Work out the finished part from the listing and answer in its coordinate system (mm). Face numbers are marked on the shaded views. A direction names the side the tool comes from. Round coordinates to 2 decimals unless told otherwise and drop trailing zeros. Loops run counter-clockwise (first coordinate to the right, second up) from the corner with the lowest first, then second, coordinate; pieces in that order, holes last. Notation, with made-up numbers: (-35, 31) - (-3, 31) arc R18 ccw to (-3, 40) - close; hole circle Ø1 at (-16, 66.25). An arc over 180 degrees is marked (long way). Use CSV: the item, a comma, the result in double quotes. Start each with the question number.
from build123d import *

# Parameters (mm, degrees)
SKETCH1_R           = 1
BOSS_EXTRUDE1_DEPTH = 1.5
CIRPATTERN1_COUNT   = 4
SKETCH3_R           = 2.525
SKETCH3_R_2         = 1.525
BOSS_EXTRUDE3_DEPTH = 7.25


with BuildPart() as part:
    # Sketch1 → Boss-Extrude1 (new body)
    with BuildSketch(Plane.XY):
        with BuildLine():
            Line((1.8, 2.706011826), (1.8, 9.915))
            ThreePointArc((1.8, 9.915), (0, 11.715), (-1.8, 9.915))
            Line((-1.8, 9.915), (-1.8, 2.706011826))
            ThreePointArc((-1.8, 2.706011826), (0, -3.25), (1.8, 2.706011826))
        make_face()
        with Locations((0, 5.015)):
            Circle(SKETCH1_R, mode=Mode.SUBTRACT)
        with Locations((0, 9.915)):
            Circle(SKETCH1_R, mode=Mode.SUBTRACT)
    boss_extrude1 = extrude(amount=BOSS_EXTRUDE1_DEPTH)

    # CirPattern1: Boss-Extrude1 ×4 about axis
    cirpattern1_axis = Axis((0, 0, 0), (0, 0, 1))
    for i in range(1, CIRPATTERN1_COUNT):
        add(boss_extrude1.rotate(cirpattern1_axis, i * 360 / CIRPATTERN1_COUNT))

    # Sketch3 → Boss-Extrude3 (add)
    # profile 1 of 3: a face of its own
    with BuildSketch(Plane.XY.offset(1.5)):
        with Locations(Location((0, 0, 0), (0, 0, 180))):
            Circle(SKETCH3_R)
        Circle(SKETCH3_R_2, mode=Mode.SUBTRACT)
    # profile 2 of 3: a face of its own
    with BuildSketch(Plane.XY.offset(1.5)):
        with BuildLine():
            ThreePointArc((1.129158979, 1.025), (0, 1.525), (-1.129158979, 1.025))
            Line((-1.129158979, 1.025), (1.129158979, 1.025))
        make_face()
    # profile 3 of 3: a face of its own
    with BuildSketch(Plane.XY.offset(1.5)):
        with BuildLine():
            ThreePointArc((1.129158979, 1.025), (0, 1.525), (-1.129158979, 1.025))
            Line((-1.129158979, 1.025), (1.129158979, 1.025))
        make_face()
    extrude(amount=BOSS_EXTRUDE3_DEPTH)


solid = part.part
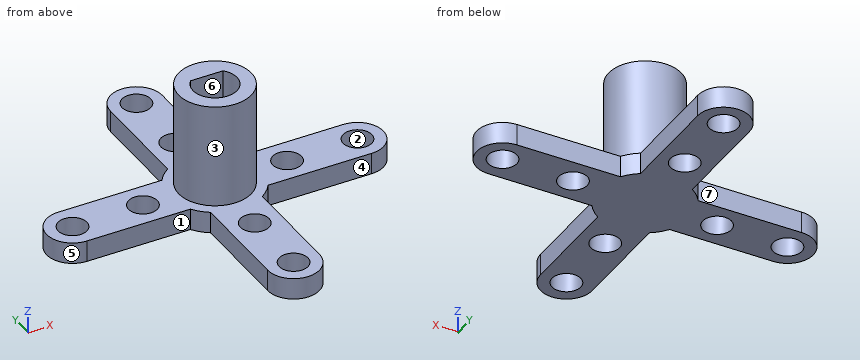
Item 1: The mould has two halves that part along Y. Classify the marked faces 5, 6 and 7: pulls with the +Y half, pulls with the -Y half, needs draft (parallel to the pull), parting line crosses it, or undercut.
Item 2: A cutting plane is placed at D-D (z = 2.5). Determine the outline of the cut face in (x, y) (3 decimals), plus the area to 3 significant figures.
Item 3: Each of these flat-tipped pins is pushed along its axis until it touches: pin 1 Ø1.6 at (x, z) = (-6, 0.5) entering from +Y; pin 2 Ø1.2 at (x, y) = (5.015, 0) entering from +Z; pin 3 Ø2.5 at (x, y) = (0, 0) entering from -Z; pin 4 Ø1.6 at (y, z) = (-7.5, 1) entering from -X. Where does it stop, or does it pass through?
Item 4: Find the intervals of material crossed by probe 1 along Y at (x, z) = (0, 1.05) (3 decimals); probe 2 along Z at (x, y) = (1.5, -9.5), in increasing order. Write a range as [from, to].
Item 5: A cutting plane is placed at A-A (y = 0). Determine the outline of the cut face in (x, z) (3 decimals), plus the area to 3 significant figures.
Item 6: A cutting plane is placed at C-C (y = 5.5). Determine the outline of the cut face in (x, z).
Item 7: Which of the six approach directions +Z, -Z, +X, -X, +Y, -Y give full straight-line access (tool end or side, diameter ignored) to the marked faces 1, 2, 3 and 4?
Item 8: A cutting plane is placed at B-B (x = 0). Determine the outline of the cut face in (y, z) (3 decimals), plus the area to 3 significant figures.
Result sheet:
1,face 5,"parting line crosses it"
1,face 6,"undercut"
1,face 7,"pulls with the +Y half"
2,outline,"circle Ø5.05 at (0, 0); hole (-1.129, 1.025) arc R1.525 ccw (long way) to (1.129, 1.025) - close"
2,area,"13.5 mm^2"
3,pin 1,"y = 1.8"
3,pin 2,"through"
3,pin 3,"z = 0"
3,pin 4,"x = -1.8"
4,probe 1,"[-11.715, -10.915], [-8.915, -6.015], [-4.015, 4.015], [6.015, 8.915], [10.915, 11.715]"
4,probe 2,"[0, 1.5]"
5,outline,"(-11.715, 0) - (-10.915, 0) - (-10.915, 1.5) - (-11.715, 1.5) - close; (-8.915, 0) - (-6.015, 0) - (-6.015, 1.5) - (-8.915, 1.5) - close; (-4.015, 0) - (4.015, 0) - (4.015, 1.5) - (2.525, 1.5) - (2.525, 8.75) - (1.525, 8.75) - (1.525, 1.5) - (-1.525, 1.5) - (-1.525, 8.75) - (-2.525, 8.75) - (-2.525, 1.5) - (-4.015, 1.5) - close; (6.015, 0) - (8.915, 0) - (8.915, 1.5) - (6.015, 1.5) - close; (10.915, 0) - (11.715, 0) - (11.715, 1.5) - (10.915, 1.5) - close"
5,area,"37.6 mm^2"
6,outline,"(-1.8, 0) - (-0.87, 0) - (-0.87, 1.5) - (-1.8, 1.5) - close; (0.87, 0) - (1.8, 0) - (1.8, 1.5) - (0.87, 1.5) - close"
7,face 1,"+Z, -Z, -X, -Y"
7,face 2,"+Z, -Z"
7,face 3,"+Z"
7,face 4,"+Z, -Z, +X, -Y"
8,outline,"(-11.715, 0) - (-10.915, 0) - (-10.915, 1.5) - (-11.715, 1.5) - close; (-8.915, 0) - (-6.015, 0) - (-6.015, 1.5) - (-8.915, 1.5) - close; (-4.015, 0) - (4.015, 0) - (4.015, 1.5) - (2.525, 1.5) - (2.525, 8.75) - (1.025, 8.75) - (1.025, 1.5) - (-1.525, 1.5) - (-1.525, 8.75) - (-2.525, 8.75) - (-2.525, 1.5) - (-4.015, 1.5) - close; (6.015, 0) - (8.915, 0) - (8.915, 1.5) - (6.015, 1.5) - close; (10.915, 0) - (11.715, 0) - (11.715, 1.5) - (10.915, 1.5) - close"
8,area,"41.3 mm^2"
